```python
from build123d import *

# Parameters (mm, degrees)
F0_W     = 1
F0_H     = 1
F0_W_2   = 2
F0_H_2   = 8
F0_W_3   = 3
F0_W_4   = 0.5
F1_DEPTH = 1.5
F2_SIZE  = 0.5


with BuildPart() as f1:
    # F0 (on Top) → F1 (new body)
    with BuildSketch(Plane.XY):
        with Locations((-2, 4.5)):
            Rectangle(F0_W, F0_H)
        with Locations((2, 4.5)):
            Rectangle(F0_W, F0_H)
        with Locations((3.5, 0)):
            Rectangle(F0_W_2, F0_H_2)
        with Locations((2, 0)):
            Rectangle(F0_W, F0_H_2)
        Rectangle(F0_W_3, F0_H_2)
        with Locations((-2, 0)):
            Rectangle(F0_W, F0_H_2)
        with Locations((-3.5, 0)):
            Rectangle(F0_W_2, F0_H_2)
        with Locations((-2, -4.5)):
            Rectangle(F0_W, F0_H)
        with Locations((2, -4.5)):
            Rectangle(F0_W, F0_H)
        with Locations((-2.75, 5.5)):
            Rectangle(F0_W_4, F0_H)
        with Locations((-2, 5.5)):
            Rectangle(F0_W, F0_H)
        with Locations((2, 5.5)):
            Rectangle(F0_W, F0_H)
        with Locations((2.75, 5.5)):
            Rectangle(F0_W_4, F0_H)
        with Locations((2, -5.5)):
            Rectangle(F0_W, F0_H)
        with Locations((2.75, -5.5)):
            Rectangle(F0_W_4, F0_H)
        with Locations((-2.75, -5.5)):
            Rectangle(F0_W_4, F0_H)
        with Locations((-2, -5.5)):
            Rectangle(F0_W, F0_H)
    extrude(amount=F1_DEPTH)

    # F2
    f2_edges = [f1.edges().sort_by_distance(p)[0] for p in [
        (-3, 6, 0.75),
        (3, 6, 0.75),
        (3, -6, 0.75),
        (-3, -6, 0.75),
    ]]
    chamfer(f2_edges, length=F2_SIZE)


solid = f1.part
```
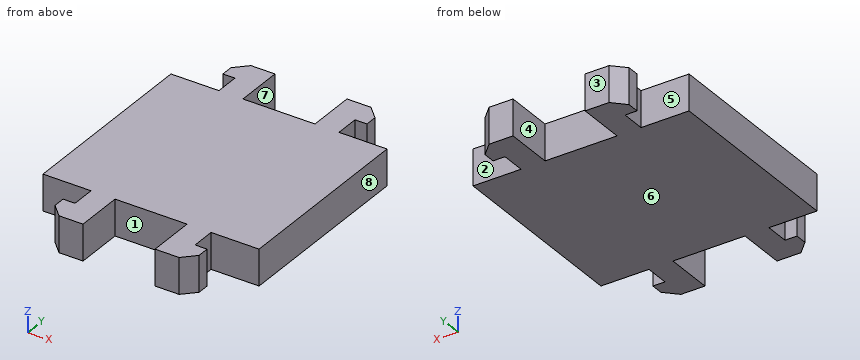
Model file for the job. Use its own axes, mm. Face numbers are marked on the shaded views. A direction names the side the tool comes from. Coordinates: 2 decimals unless noted, no trailing zeros. Order: outer loops, then holes, each group sorted by start corner. A loop starts at its lowest first (then second) coordinate and runs counter-clockwise, first axis right, second up. Notation, with made-up numbers: M 2.5,-18.75 L 25.5,-18.75 A22 ccw 25.5,20.25 Z; hole C 37,18 d6. An arc over 180 degrees is marked long. Answer as CSV lines item,"result".
(1) Band-saw the part on A-A, the plane y = -4.75. List the corners of the cut face in (x, z).
Geometry says:
outline,"M -2.5,0 L -1.5,0 L -1.5,1.5 L -2.5,1.5 Z; M 1.5,0 L 2.5,0 L 2.5,1.5 L 1.5,1.5 Z"
(2) Wall check: line 1 along X through (y, z) = (5.25, 1.4); line 2 along X through (y, z) = (-4.25, 0.45); line 3 along Y through (x, z) = (-2.75, 0.35). Give the ranges that are in metal, low to high.
Geometry says:
line 1,"x = -3 to -1.5, 1.5 to 3"
line 2,"x = -2.5 to -1.5, 1.5 to 2.5"
line 3,"y = -5.75 to -5, -4 to 4, 5 to 5.75"
(3) Flat gauge pins, fed straight in: pin 1 (0.8 mm diameter, centred on x = 3, z = 1, fed in from -Y); pin 2 (0.8 mm diameter, centred on y = -4.5, z = 0.5, fed in from +X). Where does each tip first touch, or does it go through?
Geometry says:
pin 1,"stops at y = -5.9"
pin 2,"stops at x = 2.5"
(4) Band-saw the part on C-C, the plane x = 0.5. List the corners of the cut face in (y, z), then the cut area to 3 significant figures.
Geometry says:
outline,"M -4,0 L 4,0 L 4,1.5 L -4,1.5 Z"
area,"12.0 mm2"
(5) 3-axis set-ups, long thin cutter, end or side, ignore diameter. For the marked faces 1, 2, 3, 4 and 5: which of +Z, -Z, +X, -X, +Y, -Y reach the whole face in a straight line?
Geometry says:
face 1,"+Z, -Z, -Y"
face 2,"+Z, -Z, +X"
face 3,"+Z, -Z, +X, -X, +Y"
face 4,"+Z, -Z, +Y"
face 5,"+Z, -Z, -X"
(6) Pull direction X, two halves, no side cores. Call the marked faces 6, 7 and 8: +X half, -X half, draft (parallel to the pull), parting line (faces both ways), or undercut.
Geometry says:
face 6,"draft"
face 7,"undercut"
face 8,"+X half"
